Part print with two shaded views. Sizes in mm from the minimum x, y, z corner. A direction names the side the tool comes from. Coordinates: 2 decimals unless noted, no trailing zeros. Loops run counter-clockwise (first coordinate to the right, second up) from the corner with the lowest first, then second, coordinate; pieces in that order, holes last.
(1) Slice it at A-A (z = 5). Give the cut face in (x, y), and give its area (3 significant figures).
(2) Flat gauge pins, fed straight in: P1, Ø2, axis at x = 1, y = 2.5, coming from the -Z side; P2, Ø0.5, axis at x = 3.5, y = 2.5, coming from the +Z side; P3, Ø0.6, axis at x = 3, z = 13, coming from the -Y side; P4, Ø1, axis at x = 0.5, y = 1, coming from the -Z side. Where does each tip first touch, or does it go through?
(3) Wall check: L1, parallel to Z at x = 2.5, y = 4.05; L2, parallel to X at y = 2.4, z = 12.5; L3, parallel to Z at x = 2.85, y = 0.4. Give the ranges that are in metal, low to high.
(4) Tool access for the marked faces 1 and 2: list every direction of +Z, -Z, +X, -X, +Y, -Y with a clear straight run to the whole face (end or side of a thin tool).
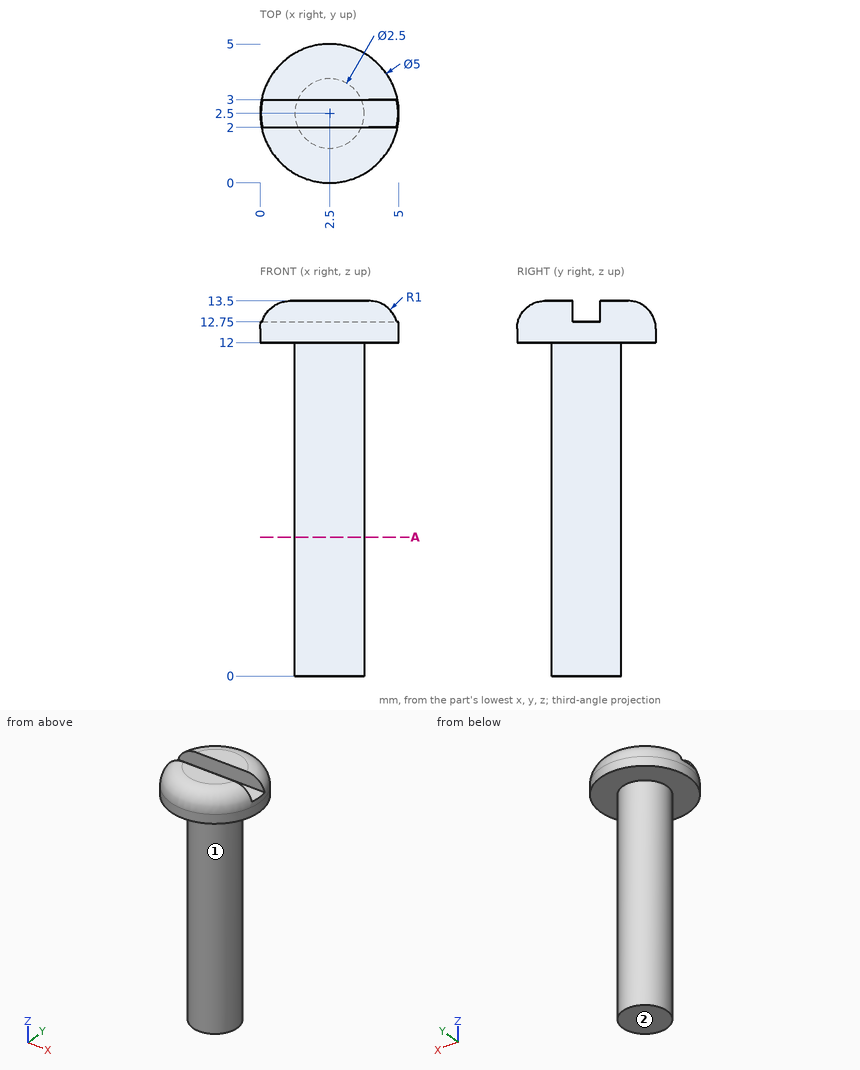
Response values:
1. outline: circle Ø2.5 at (2.5, 2.5)
1. area: 4.91 mm2
2. P1: stops at z = 0
2. P2: stops at z = 12.75
2. P3: stops at y = 0.05
2. P4: stops at z = 12
3. L1: z = 12 to 13.5
3. L2: x = 0 to 5
3. L3: z = 12 to 13.28
4. face 1: -Z
4. face 2: -Z, +X, -X, +Y, -Y
